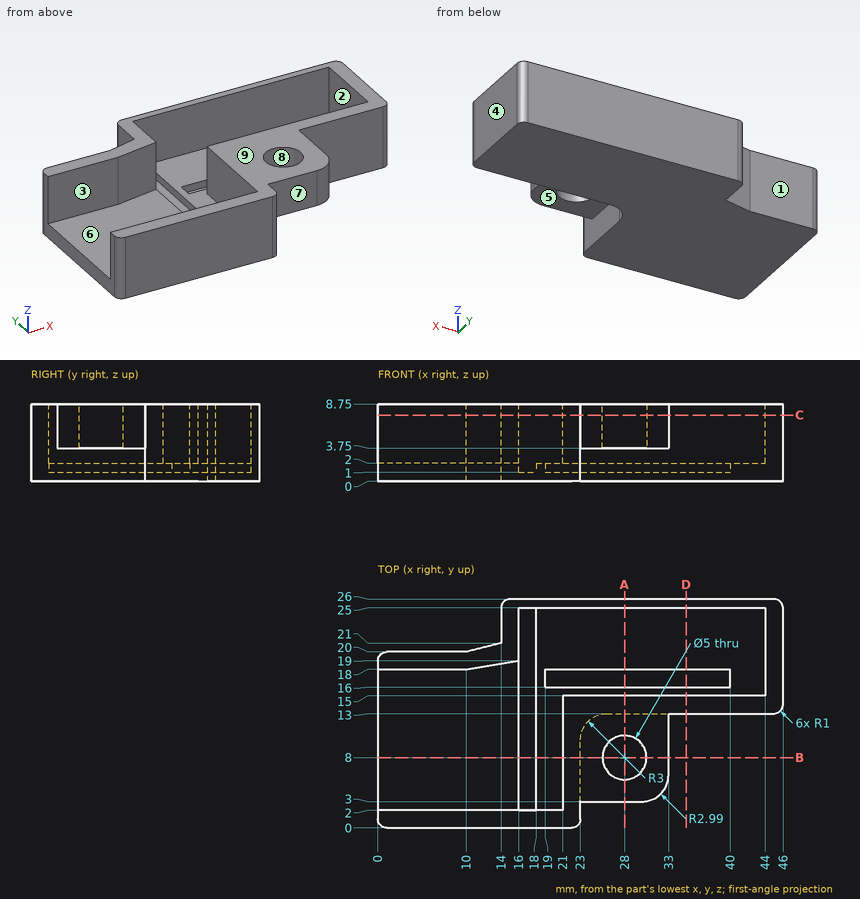
Check sheet for the drawn part. Datum: minimum x, y, z corner. Units: mm. A direction names the side the tool comes from. Give positions to 0.01 mm unless a question says otherwise; leave off trailing zeros. Order: outer loops, then holes, each group sorted by start corner. A loop starts at its lowest first (then second) coordinate and runs counter-clockwise, first axis right, second up. Notation, with made-up numbers: (4.5, 18) - (47.5, 18) arc R15 cw to (47.5, 41) - close; hole circle Ø6 at (33, 69). An arc over 180 degrees is marked (long way). Answer in a Markdown table with one row per item. Add a question column.
Q1. Material ranges on probe 1 along Y at (x, z) = (28, 7.45); probe 2 along X at (y, z) = (14, 1.75); probe 3 along X at (y, z) = (23.25, 2.25), recorded low to high. Write a range as from..to.
Q2. Cross-section at B-B, the plane y = 8. Enter the section's corners in (x, z).
Q3. Mould release check, pull along Y, two halves, no side actions. Record for the marked faces 6, 7, 8 and 9: pulls with the +Y half, pulls with the -Y half, needs draft (parallel to the pull), parting line crosses it, or undercut.
Q4. Gauge pin test, flat ends, axial feed: pin 1 (2.5 mm diameter, centred on x = 35.5, z = 4.5, fed in from -Y); pin 2 (2 mm diameter, centred on y = 14, z = 5, fed in from -X); pin 3 (6.5 mm diameter, centred on x = 28, y = 8, fed in from -Z). Record the tip position at first contact, or that the pin passes through.
Q5. Cross-section at D-D, the plane x = 35. Enter the section's corners in (y, z), then the cut area to 4 significant figures.
Q6. Cross-section at A-A, the plane x = 28. Enter the section's corners in (y, z), then the cut area to 4 significant figures.
Q7. Cross-section at C-C, the plane z = 7.5. Enter the section's corners in (x, y), then the cut area to 3 significant figures.
Q8. Tool access check on the marked faces 1, 2, 3, 4 and 5. Record the directions out of +Z, -Z, +X, -X, +Y, -Y that give a thin tool (end or side, any length) a straight path to the whole face; none if there is none.
Check values:
| question | item | result |
|---|---|---|
| 1 | probe 1 | y = 3..5.5, 10.5..15, 25..26 |
| 1 | probe 2 | x = 0..16, 18..46 |
| 1 | probe 3 | x = 14..16, 44..46 |
| 2 | outline | (0, 0) - (23, 0) - (23, 3.75) - (25.5, 3.75) - (25.5, 8.75) - (21, 8.75) - (21, 2) - (18, 2) - (18, 1) - (16, 1) - (16, 2) - (0, 2) - close; (30.5, 3.75) - (33, 3.75) - (33, 8.75) - (30.5, 8.75) - close |
| 3 | face 6 | undercut |
| 3 | face 7 | pulls with the -Y half |
| 3 | face 8 | undercut |
| 3 | face 9 | needs draft |
| 4 | pin 1 | stops at y = 13 |
| 4 | pin 2 | stops at x = 21 |
| 4 | pin 3 | stops at z = 3.75 |
| 5 | outline | (13, 0) - (26, 0) - (26, 8.75) - (25, 8.75) - (25, 2) - (18, 2) - (18, 1) - (16, 1) - (16, 2) - (15, 2) - (15, 8.75) - (13, 8.75) - close |
| 5 | area | 44.25 mm^2 |
| 6 | outline | (3, 3.75) - (5.5, 3.75) - (5.5, 8.75) - (3, 8.75) - close; (10.5, 3.75) - (13, 3.75) - (13, 0) - (26, 0) - (26, 8.75) - (25, 8.75) - (25, 2) - (18, 2) - (18, 1) - (16, 1) - (16, 2) - (15, 2) - (15, 8.75) - (10.5, 8.75) - close |
| 6 | area | 69.25 mm^2 |
| 7 | outline | (0, 1) arc R1 ccw to (1, 0) - (22, 0) arc R1 ccw to (23, 1) - (23, 3) - (30.01, 3) arc R2.99 ccw to (33, 5.99) - (33, 13) - (45, 13) arc R1 ccw to (46, 14) - (46, 25) arc R1 ccw to (45, 26) - (15, 26) arc R1 ccw to (14, 25) - (14, 21) - (10, 20) - (1, 20) arc R1 ccw to (0, 19) - (0, 18) - (10, 18) - (16, 19) - (16, 25) - (44, 25) - (44, 15) - (21, 15) - (21, 2) - (0, 2) - close; hole circle Ø5 at (28, 8) |
| 7 | area | 288 mm^2 |
| 8 | face 1 | +Z, -Z, -X, +Y |
| 8 | face 2 | +Z |
| 8 | face 3 | +Z, -X |
| 8 | face 4 | +Z, -Z, +X, +Y, -Y |
| 8 | face 5 | -Z, +X, -Y |
